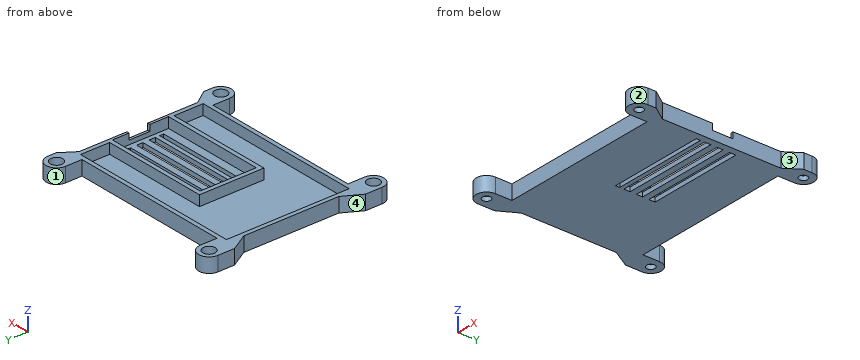
from build123d import *

# Parameters (mm, degrees)
EXTRUDE_1_DEPTH     = 2
SKETCH_3_W          = 50
SKETCH_3_H          = 27
EXTRUDE_2_DEPTH     = 5
SKETCH_5_R          = 3
CUT_EXTRUDE_1_DEPTH = 5
SKETCH_6_W          = 3
SKETCH_6_H          = 10
CUT_EXTRUDE_2_DEPTH = 102.540368708
CUT_EXTRUDE_START   = -7
CUT_EXTRUDE_5_DEPTH = 7
SKETCH_9_W          = 83.2
SKETCH_9_H          = 14.002207555
SKETCH_9_W_2        = 32
SKETCH_9_H_2        = 31
CUT_EXTRUDE_6_DEPTH = 5
SKETCH_11_W         = 46
SKETCH_11_H         = 3
SKETCH_11_H_2       = 2
CUT_EXTRUDE_8_DEPTH = 10
SKETCH_14_R         = 2
CUT_EXTRUDE_9_DEPTH = 10


# Read off the part's stored shape, not the designer's step: the extrude step
with BuildPart() as part:
    # 草图1 → 凸台-拉伸1 (new body)
    with BuildSketch(Plane.XY):
        with BuildLine():
            Line((-46, 22.841953517), (-46, -22.841953517))
            Line((-46, -22.841953517), (-51, -31.502207555))
            Line((-51, -31.502207555), (-51, -39.502207555))
            ThreePointArc((-51, -39.502207555), (-46, -44.502207555), (-41, -39.502207555))
            Line((-41, -39.502207555), (-41, -31.502207555))
            Line((-41, -31.502207555), (36, -31.502207555))
            Line((36, -31.502207555), (36, -39.502207555))
            ThreePointArc((36, -39.502207555), (41, -44.502207555), (46, -39.502207555))
            Line((46, -39.502207555), (46, 39.502207555))
            ThreePointArc((46, 39.502207555), (41, 44.502207555), (36, 39.502207555))
            Line((36, 39.502207555), (36, 31.502207555))
            Line((36, 31.502207555), (-41, 31.502207555))
            Line((-41, 31.502207555), (-41, 39.502207555))
            ThreePointArc((-41, 39.502207555), (-46, 44.502207555), (-51, 39.502207555))
            Line((-51, 39.502207555), (-51, 31.502207555))
            Line((-51, 31.502207555), (-46, 22.841953517))
        make_face()
    extrude(amount=EXTRUDE_1_DEPTH)

    # 草图3 → 凸台-拉伸2 (add)
    with BuildSketch(Plane.XY.offset(2)):
        with BuildLine():
            Line((-51, 39.502207555), (-51, 31.502207555))
            Line((-51, 31.502207555), (-46, 22.841953517))
            Line((-46, 22.841953517), (-46, -22.841953517))
            Line((-46, -22.841953517), (-51, -31.502207555))
            Line((-51, -31.502207555), (-51, -39.502207555))
            ThreePointArc((-51, -39.502207555), (-46, -44.502207555), (-41, -39.502207555))
            Line((-41, -39.502207555), (-41, -31.502207555))
            Line((-41, -31.502207555), (36, -31.502207555))
            Line((36, -31.502207555), (36, -39.502207555))
            ThreePointArc((36, -39.502207555), (41, -44.502207555), (46, -39.502207555))
            Line((46, -39.502207555), (46, 39.502207555))
            ThreePointArc((46, 39.502207555), (41, 44.502207555), (36, 39.502207555))
            Line((36, 39.502207555), (36, 31.502207555))
            Line((36, 31.502207555), (-41, 31.502207555))
            Line((-41, 31.502207555), (-41, 39.502207555))
            ThreePointArc((-41, 39.502207555), (-46, 44.502207555), (-51, 39.502207555))
        make_face()
        with Locations((15, 0)):
            Rectangle(SKETCH_3_W, SKETCH_3_H, mode=Mode.SUBTRACT)
    extrude(amount=EXTRUDE_2_DEPTH)

    # 草图5 → 切除-拉伸1 (cut)
    with BuildSketch(Plane.XY.offset(7)):
        with Locations((41, 39.502207555)):
            Circle(SKETCH_5_R)
        with Locations((-46, 39.502207555)):
            Circle(SKETCH_5_R)
        with Locations((41, -39.502207555)):
            Circle(SKETCH_5_R)
        with Locations((-46, -39.502207555)):
            Circle(SKETCH_5_R)
    extrude(amount=-CUT_EXTRUDE_1_DEPTH, mode=Mode.SUBTRACT)

    # 草图6 → 切除-拉伸2 (cut, through all)
    with BuildSketch(Plane.ZY.offset(-40)):
        with Locations((5.5, 0.5)):
            Rectangle(SKETCH_6_W, SKETCH_6_H)
    extrude(amount=-CUT_EXTRUDE_2_DEPTH, mode=Mode.SUBTRACT)

    # 切除-拉伸5 outline → 切除-拉伸5 (cut)
    with BuildSketch(Plane.XY.offset(7).offset(CUT_EXTRUDE_START)):
        Polygon((46, 35.502207555), (41.2, 28.502207555), (41.2, -28.502207555), (46, -35.502207555), align=None)
    extrude(amount=CUT_EXTRUDE_5_DEPTH, mode=Mode.SUBTRACT)

    # 草图9 → 切除-拉伸6 (cut)
    with BuildSketch(Plane.XY.offset(7)):
        with Locations((-2.4, 22.501103778)):
            Rectangle(SKETCH_9_W, SKETCH_9_H)
        with Locations((-2.4, -22.501103778)):
            Rectangle(SKETCH_9_W, SKETCH_9_H)
        with Locations((-28, 0)):
            Rectangle(SKETCH_9_W_2, SKETCH_9_H_2)
    extrude(amount=-CUT_EXTRUDE_6_DEPTH, mode=Mode.SUBTRACT)

    # 草图11 → 切除-拉伸8 (cut)
    with BuildSketch(Plane.XY.offset(2)):
        with Locations((15, 8)):
            Rectangle(SKETCH_11_W, SKETCH_11_H)
        with Locations((15, 2)):
            Rectangle(SKETCH_11_W, SKETCH_11_H)
        with Locations((15, -4)):
            Rectangle(SKETCH_11_W, SKETCH_11_H)
        with Locations((15, -8.5)):
            Rectangle(SKETCH_11_W, SKETCH_11_H_2)
    extrude(amount=-CUT_EXTRUDE_8_DEPTH, mode=Mode.SUBTRACT)

    # 草图14 → 切除-拉伸9 (cut)
    with BuildSketch(Plane.XY.offset(2)):
        with Locations((41, -39.502207555)):
            Circle(SKETCH_14_R)
        with Locations((41, 39.502207555)):
            Circle(SKETCH_14_R)
        with Locations((-46, 39.502207555)):
            Circle(SKETCH_14_R)
        with Locations((-46, -39.502207555)):
            Circle(SKETCH_14_R)
    extrude(amount=-CUT_EXTRUDE_9_DEPTH, mode=Mode.SUBTRACT)


solid = part.part
The model under review builds one solid part; all positions refer to its coordinate system, in mm. Face numbers are marked on the shaded views. Round coordinates to 2 decimals unless told otherwise and drop trailing zeros. Write each loop counter-clockwise with the first axis right and the second up, starting at its lowest first coordinate (ties: lowest second). Pieces come first, ordered by that corner, then holes. Notation, with made-up numbers: M 79,51.5 L 131,51.5 A24 cw 131,76.5 Z; hole C 45,45 d5. An arc over 180 degrees is marked long. Answer as CSV lines item,"result". Start each with the question number.
Q1. The part is to be moulded in two halves that separate along X. For the marked faces 1, 2, 3 and 4, say which applies: +X half, -X half, draft (parallel to the pull), parting line (faces both ways), or undercut.
Q2. Consider section D-D, the plane y = -33.5. Give the boundary of the cut face in (x, z), then the cut area to 3 significant figures.
Q3. Clearance check with flat-ended pins moving along their axes: P1, Ø5, axis at x = 7.5, y = -12.5, coming from the +Z side; P2, Ø4, axis at x = 14.5, z = 1, coming from the +Y side; P3, Ø1.5, axis at x = 18, z = 1.5, coming from the -Y side; P4, Ø2, axis at y = 9, z = 5, coming from the +X side. State where each tip first meets the part, or that it passes through.
Q4. Consider section A-A, the plane x = 28. State how many separate pieces and enclosed holes the cut face has, then the cut area to 3 significant figures.
Q5. Consider section B-B, the plane y = 11.5. Give the boundary of the cut face in (x, z), then the cut area to 3 significant figures.
Q6. Wall thickness on line 1 along X through (y, z) = (6, 2.5); line 2 along Y through (x, z) = (2, 6); line 3 along Y through (x, z) = (-5.5, 1.5): over which ranges is each line inside the solid? List them lowest first.
Result set:
1,face 1,"undercut"
1,face 2,"undercut"
1,face 3,"+X half"
1,face 4,"-X half"
2,outline,"M -51,0 L -41,0 L -41,7 L -51,7 Z; M 36,0 L 44.63,0 L 44.63,7 L 36,7 Z"
2,area,"130 mm²"
3,P1,"stops at z = 7"
3,P2,"stops at y = 31.5"
3,P3,"stops at y = -31.5"
3,P4,"stops at x = 41.2"
4,separate pieces,"5"
4,enclosed holes,"0"
4,area,"144 mm²"
5,outline,"M -46,0 L 41.2,0 L 41.2,7 L 40,7 L 40,2 L -10,2 L -10,7 L -12,7 L -12,2 L -44,2 L -44,7 L -46,7 Z"
5,area,"200 mm²"
6,line 1,"x = -46 to -44, -12 to -10, 40 to 41.2"
6,line 2,"y = -31.5 to -29.5, -15.5 to -13.5, 13.5 to 15.5, 29.5 to 31.5"
6,line 3,"y = -31.5 to -9.5, -7.5 to -5.5, -2.5 to 0.5, 3.5 to 6.5, 9.5 to 31.5"
